Work out the finished part from the listing and answer in its coordinate system (mm). Face numbers are marked on the shaded views. A direction names the side the tool comes from. Give positions to 0.01 mm unless a question says otherwise; leave off trailing zeros. Loops run counter-clockwise (first coordinate to the right, second up) from the corner with the lowest first, then second, coordinate; pieces in that order, holes last. Notation, with made-up numbers: M -6.5,51.25 L 17.5,51.25 A29 ccw 17.5,77.25 Z; hole C 39,42.5 d2. An arc over 180 degrees is marked long. Use a Markdown table: item, result.
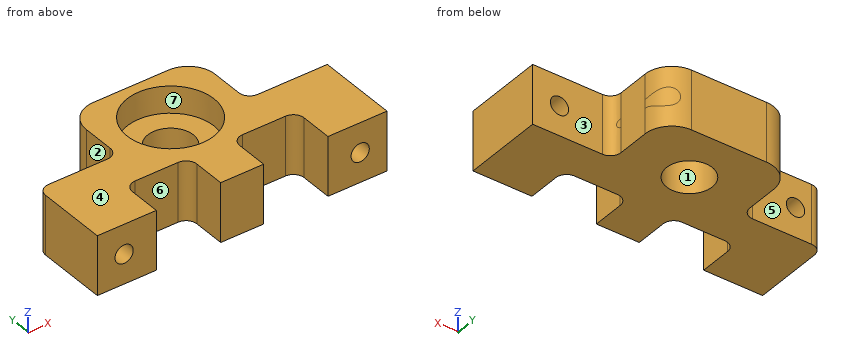
```python
from build123d import *

# Parameters (mm, degrees)
SKETCH_1_W               = 24
SKETCH_1_H               = 28
SKETCH_1_R               = 4.25
EXTRUDE_1_DEPTH          = 11
SKETCH_2_R               = 8.1
CUT_EXTRUDE_1_DEPTH      = 5
SKETCH_6_W               = 15
SKETCH_6_H               = 15
EXTRUDE_2_DEPTH          = 11
CUT_EXTRUDE_3_DEPTH      = 33.787192622
CUT_EXTRUDE_3_DEPTH_BACK = 33.787192622
SKETCH_7_R               = 1.7
SKETCH_8_W               = 12
SKETCH_8_H               = 8
CUT_EXTRUDE_4_DEPTH      = 33.341923258
FILLET_1_R               = 2
FILLET_2_R               = 2
FILLET_3_R               = 5
SKETCH_9_R               = 1.7
EXTRUDE_3_DEPTH          = 25
CUT_EXTRUDE_5_DEPTH      = 25


with BuildPart() as part:
    # 草图1 → 凸台-拉伸1 (new body)
    with BuildSketch(Plane.XY):
        Rectangle(SKETCH_1_W, SKETCH_1_H)
        with Locations((0, 4)):
            Circle(SKETCH_1_R, mode=Mode.SUBTRACT)
    extrude(amount=EXTRUDE_1_DEPTH)

    # 草图2 → 切除-拉伸1 (cut)
    with BuildSketch(Plane.XY.offset(11)):
        with Locations((0, 4)):
            Circle(SKETCH_2_R)
    extrude(amount=-CUT_EXTRUDE_1_DEPTH, mode=Mode.SUBTRACT)

    # 草图6 → 凸台-拉伸2 (add)
    with BuildSketch(Plane.XY.offset(11)):
        with Locations((-19.5, -6.5)):
            Rectangle(SKETCH_6_W, SKETCH_6_H)
        with Locations((19.5, -6.5)):
            Rectangle(SKETCH_6_W, SKETCH_6_H)
    extrude(amount=-EXTRUDE_2_DEPTH)

    # 草图7 → 切除-拉伸3 (cut, two sides: drawn at the far end of the back side and taken through both)
    with BuildSketch(Plane(origin=(0, 1, 0), x_dir=(1, 0, 0), z_dir=(0, 1, 0)).offset(-CUT_EXTRUDE_3_DEPTH_BACK)):
        with Locations(Location((22, -5.5, 0), (0, 0, 180))):
            Circle(SKETCH_7_R)
        with Locations(Location((-22, -5.5, 0), (0, 0, 180))):
            Circle(SKETCH_7_R)
        with Locations(Location((10.5, -5.5, 0), (0, 0, 180))):
            Circle(SKETCH_7_R)
    extrude(amount=CUT_EXTRUDE_3_DEPTH + CUT_EXTRUDE_3_DEPTH_BACK, mode=Mode.SUBTRACT)

    # 草图8 → 切除-拉伸4 (cut, through all)
    with BuildSketch(Plane.XY.offset(11)):
        with Locations((-10, -10)):
            Rectangle(SKETCH_8_W, SKETCH_8_H)
        with Locations((10, -10)):
            Rectangle(SKETCH_8_W, SKETCH_8_H)
    extrude(amount=-CUT_EXTRUDE_4_DEPTH, mode=Mode.SUBTRACT)

    # 圆角1
    fillet_1_edges = [part.edges().sort_by_distance(p)[0] for p in [
        (-16, -6, 5.5),
        (-4, -6, 5.5),
        (4, -6, 5.5),
        (16, -6, 5.5),
    ]]
    fillet(fillet_1_edges, radius=FILLET_1_R)

    # 圆角2
    # the kernel refuses this fillet: 2 mm, written as the material it adds along each edge
    with BuildSketch(Plane(origin=(12, 1, 11), x_dir=(1, 0, 0), z_dir=(0, 0, -1))) as fillet_2_piece_1_section:
        with BuildLine():
            CenterArc((FILLET_2_R, -FILLET_2_R), FILLET_2_R, 90, 90)
            Line((0, -FILLET_2_R), (0, 0))
            Line((0, 0), (FILLET_2_R, 0))
        make_face()
    fillet_2_piece_1 = extrude(amount=9.7, mode=Mode.PRIVATE)
    fillet_2_piece_1 = fillet_2_piece_1 - Plane(origin=(10.5, 1.435440369, 5.5), x_dir=(-1, 0, 0), z_dir=(0, -1, 0)) * Cylinder(1.7, 28, mode=Mode.PRIVATE)
    add(fillet_2_piece_1)
    with BuildSketch(Plane(origin=(12, 1, 9.7), x_dir=(0, 1, 0), z_dir=(0, 0, -1))) as fillet_2_piece_2_section:
        with BuildLine():
            CenterArc((FILLET_2_R, FILLET_2_R), FILLET_2_R, 180, 90)
            Line((0, FILLET_2_R), (0, 0))
            Line((0, 0), (FILLET_2_R, 0))
        make_face()
    fillet_2_piece_2 = extrude(amount=9.7, mode=Mode.PRIVATE)
    fillet_2_piece_2 = fillet_2_piece_2 - Plane(origin=(10.5, 1.435440365, 5.5), x_dir=(-1, 0, 0), z_dir=(0, -1, 0)) * Cylinder(1.7, 28, mode=Mode.PRIVATE)
    add(fillet_2_piece_2)
    with BuildSketch(Plane(origin=(-12, 1, 11), x_dir=(-1, 0, 0), z_dir=(0, 0, -1))) as fillet_2_piece_3:
        with BuildLine():
            CenterArc((FILLET_2_R, FILLET_2_R), FILLET_2_R, 180, 90)
            Line((0, FILLET_2_R), (0, 0))
            Line((0, 0), (FILLET_2_R, 0))
        make_face()
    extrude(amount=11)
    # the kernel refuses this fillet: 2 mm, written as the material it takes off along each edge
    with BuildSketch(Plane(origin=(-27, 1, 16), x_dir=(0, -1, 0), z_dir=(0, 0, -1))) as fillet_2_2_piece_1:
        with BuildLine():
            CenterArc((FILLET_2_R, -FILLET_2_R), FILLET_2_R, 90, 90)
            Line((0, -FILLET_2_R), (0, 0))
            Line((0, 0), (FILLET_2_R, 0))
        make_face()
    extrude(amount=21, mode=Mode.SUBTRACT)

    # 圆角3
    # the kernel refuses this fillet: 5 mm, written as the material it takes off along each edge
    with BuildSketch(Plane(origin=(12, 14, -6.2), x_dir=(-1, 0, 0), z_dir=(0, 0, 1))) as fillet_3_piece_1:
        with BuildLine():
            CenterArc((FILLET_3_R, FILLET_3_R), FILLET_3_R, 180, 90)
            Line((0, FILLET_3_R), (0, 0))
            Line((0, 0), (FILLET_3_R, 0))
        make_face()
    extrude(amount=29.7, mode=Mode.SUBTRACT)
    with BuildSketch(Plane(origin=(-12, 14, -12.5), x_dir=(0, -1, 0), z_dir=(0, 0, 1))) as fillet_3_piece_2:
        with BuildLine():
            CenterArc((FILLET_3_R, FILLET_3_R), FILLET_3_R, 180, 90)
            Line((0, FILLET_3_R), (0, 0))
            Line((0, 0), (FILLET_3_R, 0))
        make_face()
    extrude(amount=36, mode=Mode.SUBTRACT)

    # 草图9 → 凸台-拉伸3 (add)
    with BuildSketch(Plane.XZ.offset(6)):
        with Locations((10.5, 5.5)):
            Circle(SKETCH_9_R)
    extrude(amount=-EXTRUDE_3_DEPTH)

    # 草图10 → 切除-拉伸5 (cut)
    with BuildSketch(Plane.XY.offset(11)):
        with BuildLine():
            Line((12, 3), (12, 9))
            ThreePointArc((12, 9), (10.535533906, 12.535533906), (7, 14))
            Line((7, 14), (7.594175957, 21.794622096))
            Line((7.594175957, 21.794622096), (15.452945432, 21.794622096))
            Line((15.452945432, 21.794622096), (16.462328667, 6.870169973))
            Line((16.462328667, 6.870169973), (14, 1))
            ThreePointArc((14, 1), (12.585786438, 1.585786438), (12, 3))
        make_face()
    extrude(amount=-CUT_EXTRUDE_5_DEPTH, mode=Mode.SUBTRACT)


solid = part.part
```
(1) The mould has two halves that part along Y. Classify the marked faces 1, 2 and 3: released by +Y, released by -Y, zero draft, split by the parting line, or undercut.
Entries:
| item | result |
|---|---|
| face 1 | undercut |
| face 2 | zero draft |
| face 3 | released by +Y |
(2) Which of the six approach directions +Z, -Z, +X, -X, +Y, -Y give full straight-line access (tool end or side, diameter ignored) to the marked faces 4, 5, 6 and 7?
Entries:
| item | result |
|---|---|
| face 4 | +Z, +X, -X, +Y, -Y |
| face 5 | +Z, -Z, -X, +Y |
| face 6 | +Z, -Z, -Y |
| face 7 | +Z |
(3) A cutting plane is placed at C-C (z = 8.25). Write down the section's boundary in (x, y), and give its area (3 significant figures).
Entries:
| item | result |
|---|---|
| outline | M -27,-14 L -16,-14 L -16,-8 A2 cw -14,-6 L -6,-6 A2 cw -4,-8 L -4,-14 L 4,-14 L 4,-8 A2 cw 6,-6 L 14,-6 A2 cw 16,-8 L 16,-14 L 27,-14 L 27,1 L 14,1 A2 cw 12,3 L 12,9 A5 ccw 7,14 L -7,14 A5 ccw -12,9 L -12,3 A2 cw -14,1 L -25,1 A2 ccw -27,-1 Z; hole C 0,4 d16.2 |
| area | 717 mm² |
(4) A cutting plane is placed at D-D (z = 5.5). Count the separate pieces of the cut face and the enclosed holes in it, and give its area (3 significant figures).
Entries:
| item | result |
|---|---|
| separate pieces | 3 |
| enclosed holes | 1 |
| area | 765 mm² |
(5) A cutting plane is placed at B-B (x = 0). Write down the section's boundary in (y, z), and give its area (3 significant figures).
Entries:
| item | result |
|---|---|
| outline | M -14,0 L -0.25,0 L -0.25,6 L -4.1,6 L -4.1,11 L -14,11 Z; M 8.25,0 L 14,0 L 14,11 L 12.1,11 L 12.1,6 L 8.25,6 Z |
| area | 176 mm² |
(6) A cutting plane is placed at A-A (y = -8.5). Write down the section's boundary in (x, z), and give its area (3 significant figures).
Entries:
| item | result |
|---|---|
| outline | M -27,0 L -16,0 L -16,11 L -27,11 Z; M -4,0 L 4,0 L 4,11 L -4,11 Z; M 16,0 L 27,0 L 27,11 L 16,11 Z; hole C -22,5.5 d3.4; hole C 22,5.5 d3.4 |
| area | 312 mm² |
(7) Consider probe 1 along X at (y, z) = (-3.25, 5.5); probe 2 along X at (y, z) = (-9.5, 5.5); probe 3 along Z at (x, y) = (22, -5.25). Determine where each line is inside the solid, lowest interval first. Write a range as [from, to].
Entries:
| item | result |
|---|---|
| probe 1 | x = [-27, -23.7], [-20.3, 20.3], [23.7, 27] |
| probe 2 | x = [-27, -23.7], [-20.3, -16], [-4, 4], [16, 20.3], [23.7, 27] |
| probe 3 | z = [0, 3.8], [7.2, 11] |
(8) Given P1, Ø4, axis at x = 9, z = 5, coming from the -Y side; P2, Ø4, axis at y = 10, z = 3.5, coming from the +X side; P3, Ø5, axis at y = 7, z = 6, coming from the -X side, each flat-ended and moving along its own axis, determine where each tip first touches the part or whether it passes through.
Entries:
| item | result |
|---|---|
| P1 | stops at y = -6 |
| P2 | stops at x = 12 |
| P3 | stops at x = -12 |
